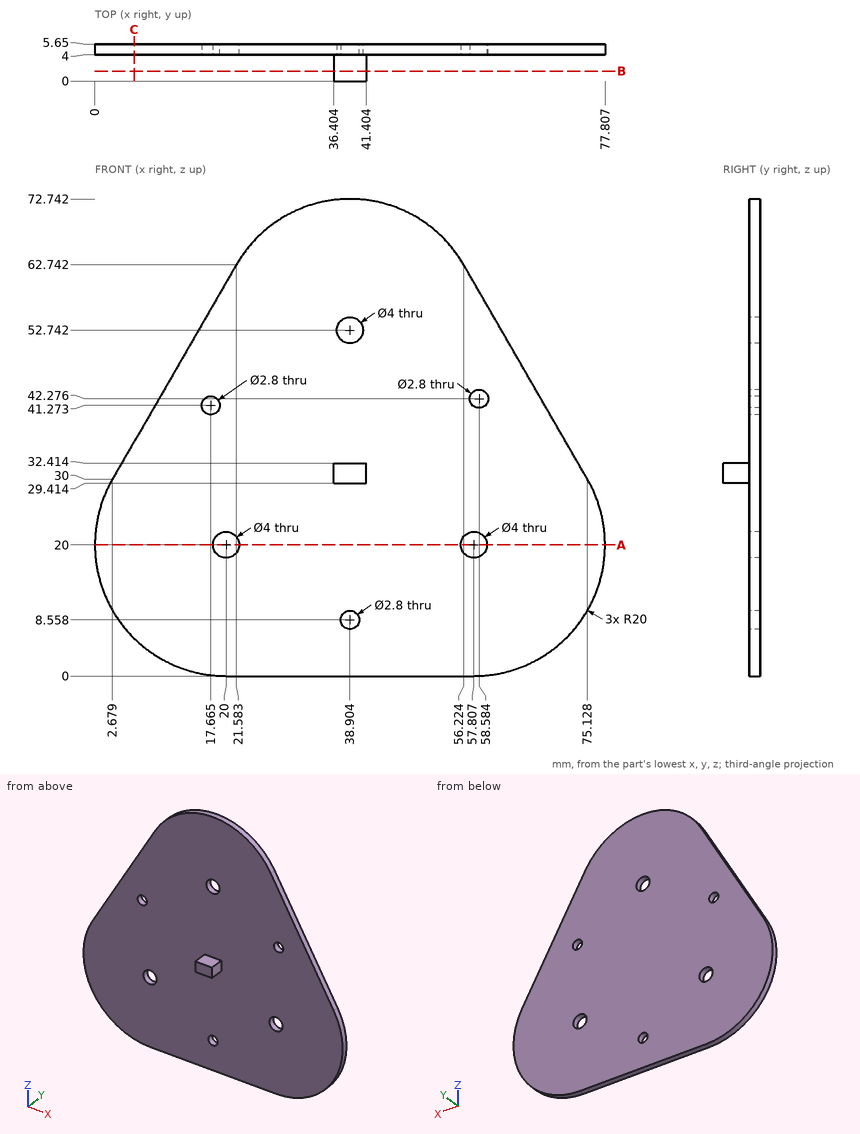
Here's the drawing with two shaded views (mm, measured from the low corner). I have some questions. Give positions to 0.01 mm unless a question says otherwise; leave off trailing zeros. Loops run counter-clockwise (first coordinate to the right, second up) from the corner with the lowest first, then second, coordinate; pieces in that order, holes last. Notation, with made-up numbers: M 34,65 L 93,65 A26 cw 93,92 Z; hole C 44.5,86.5 d4. An arc over 180 degrees is marked long. Use one line per item in the form item = value. Start each with the question number.
Q1. Will these pins go through, and if not, where does the flat tip stop? pin 1 Ø3 at (x, z) = (38.9, 8.56) entering from -Y; pin 2 Ø1.5 at (y, z) = (2, 31) entering from +X; pin 3 Ø2 at (x, y) = (40, 1.5) entering from -Z.
Q2. If we section it at C-C (x = 6): Write out the boundary of the cut face in (y, z).
Q3. If we section it at B-B (y = 1.5): Write out the boundary of the cut face in (x, z), then the cut area to 3 significant figures.
Q4. I need wall thicknesses on line 1 along X through (y, z) = (4.5, 42.5) (1 decimal); line 2 along Y through (x, z) = (69, 39.5); line 3 along Z through (x, y) = (37, 3.7). Which ranges of each line are inside material? Lowest first, please.
Q5. If we section it at A-A (z = 20): Write out the boundary of the cut face in (x, y).
Taken from the geometry:
q1.pin_1 = 4
q1.pin_2 = 41.4
q1.pin_3 = 29.41
q2.outline = M 4,5.72 L 5.65,5.72 L 5.65,35.75 L 4,35.75 Z
q3.outline = M 36.4,29.41 L 41.4,29.41 L 41.4,32.41 L 36.4,32.41 Z
q3.area = 15.0 mm^2
q4.line_1 = 9.9 to 17, 18.3 to 57.2, 60 to 67.9
q4.line_2 = 4 to 5.65
q4.line_3 = 29.41 to 32.41
q5.outline = M 0,4 L 18,4 L 18,5.65 L 0,5.65 Z; M 22,4 L 55.81,4 L 55.81,5.65 L 22,5.65 Z; M 59.81,4 L 77.81,4 L 77.81,5.65 L 59.81,5.65 Z
